Verification items for this drawing (mm, ordinates from the low corner). A direction names the side the tool comes from. Round coordinates to 2 decimals unless told otherwise and drop trailing zeros. Order: outer loops, then holes, each group sorted by start corner. A loop starts at its lowest first (then second) coordinate and runs counter-clockwise, first axis right, second up. Notation, with made-up numbers: M -32.5,39 L 22.5,39 A23 ccw 22.5,59 Z; hole C 42,13 d1. An arc over 180 degrees is marked long. Use CSV: the item, a comma, the result in double quotes. Start each with the question number.
Q1. Sectioned sample at A-A (x = 14). Enter the section's corners in (y, z), and give its area (3 significant figures).
Q2. Sectioned sample at B-B (y = 24.5). Enter the section's corners in (x, z), and give its area (4 significant figures).
Q3. Set-up check for the marked faces 1 and 2: record each of +Z, -Z, +X, -X, +Y, -Y from which the full face is reachable in a straight line by a thin tool's end or side.
Q4. Scan lines: line 1 (Z direction, x = 37, y = 21.5); line 2 (X direction, y = 19, z = 1); line 3 (Y direction, x = 51.5, z = 10.75). Record each from-to range of solid material in increasing order.
Q5. Gauge pin test, flat ends, axial feed: pin 1 Ø1.2 at (y, z) = (10.5, 10) entering from +X; pin 2 Ø5.5 at (x, z) = (8, 2) entering from -Y; pin 3 Ø1 at (x, y) = (44.5, 22) entering from -Z; pin 4 Ø1 at (y, z) = (6.5, 3.5) entering from +X. Record the tip position at first contact, or that the pin passes through.
Q6. Sectioned sample at C-C (z = 1.5). Enter the section's corners in (x, y).
Q7. Sectioned sample at D-D (y = 13). Enter the section's corners in (x, z), and give its area (3 significant figures).
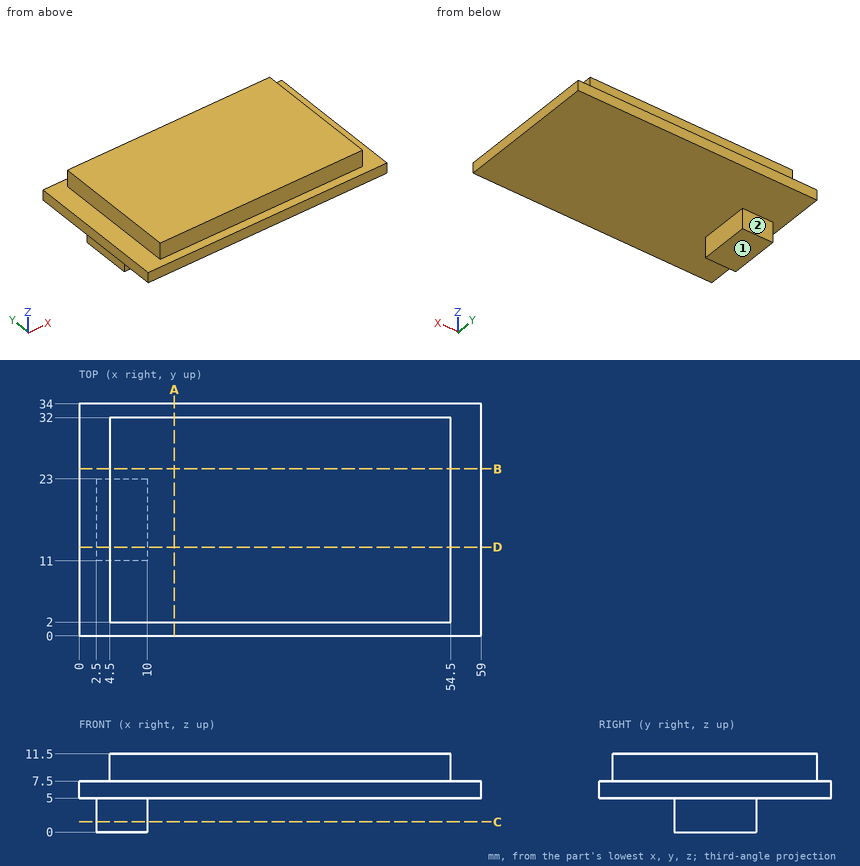
Verdict:
1,outline,"M 0,5 L 34,5 L 34,7.5 L 32,7.5 L 32,11.5 L 2,11.5 L 2,7.5 L 0,7.5 Z"
1,area,"205 mm²"
2,outline,"M 0,5 L 59,5 L 59,7.5 L 54.5,7.5 L 54.5,11.5 L 4.5,11.5 L 4.5,7.5 L 0,7.5 Z"
2,area,"347.5 mm²"
3,face 1,"-Z, +X, -X, +Y, -Y"
3,face 2,"-Z, +X, -X, +Y"
4,line 1,"z = 5 to 11.5"
4,line 2,"x = 2.5 to 10"
4,line 3,"y = 2 to 32"
5,pin 1,"stops at x = 54.5"
5,pin 2,"stops at y = 11"
5,pin 3,"stops at z = 5"
5,pin 4,"passes through"
6,outline,"M 2.5,11 L 10,11 L 10,23 L 2.5,23 Z"
7,outline,"M 0,5 L 2.5,5 L 2.5,0 L 10,0 L 10,5 L 59,5 L 59,7.5 L 54.5,7.5 L 54.5,11.5 L 4.5,11.5 L 4.5,7.5 L 0,7.5 Z"
7,area,"385 mm²"
